Geometry: final body of the model. Coordinates: model frame, mm. A direction names the side the tool comes from. Give positions to 0.01 mm unless a question says otherwise; leave off trailing zeros. Write each loop counter-clockwise with the first axis right and the second up, starting at its lowest first coordinate (ties: lowest second). Pieces come first, ordered by that corner, then holes. Notation, with made-up numbers: (-15, 82) -> (0, 82) arc R32 cw to (0, 115) -> close; hole circle Ø3 at (17.5, -33). An arc over 180 degrees is marked (long way). Answer as a JSON object with one key per item and string values. Group by question number.
(1) Section query A-A on x = 6.75. Output: boundary loops of the cut face in (y, z), plus the area to 3 significant figures.
(2) Draft query along Y for faces 6 (the face through (12.32, -14.79, 61.76)), 7 (the face through (12, -6, 50)), 8 (the face through (12, -45, 140)). Return one class per face: +Y half, -Y half, draft (parallel to the pull), parting line (faces both ways), or undercut.
(3) Material intervals for probe 1 along Z at (x, y) = (13.5, -53.5); probe 2 along X at (y, z) = (-6, 33); probe 3 along Y at (x, z) = (12.5, 38.5), sorted ascending.
(4) Section query C-C on x = 22.5. Output: boundary loops of the cut face in (y, z), plus the area to 3 significant figures.
(5) Set-up query: faces 1 (the face through (6, -45, 110)), 2 (the face through (12, -53, 25)), 3 (the face through (12, 0, 26)), 4 (the face through (0, -37, 56)), 5 (the face through (12, -30, 105)). Return all of +Z, -Z, +X, -X, +Y, -Y with unobstructed straight access to the full face (end or side cutting, diameter ignored); none if empty.
(6) Contact query for flat-ended pins moving along their axis: pin 1 Ø12.5 at (x, z) = (17, 116.5) entering from +Y; pin 2 Ø7 at (x, y) = (12.5, -6) entering from +Z; pin 3 Ø8 at (x, y) = (2.5, -13) entering from +Z. Output: stop coordinate, or through.
(7) Section query B-B on y = -25. Output: boundary loops of the cut face in (x, z), plus the area to 3 significant figures.
(8) Section query D-D on y = -13. Output: boundary loops of the cut face in (x, z).
from build123d import *

# Parameters (mm, degrees)
F1_DEPTH = 25
F3_DEPTH = 50
F5_DEPTH = 60


with BuildPart() as f1:
    # F0 (on Right) → F1 (new body)
    with BuildSketch(Plane.YZ):
        with BuildLine():
            Line((-60, 0), (0, 0))
            Line((0, 0), (0, 53.749684))
            Line((0, 53.749684), (-30, 70))
            Line((-30, 70), (-30, 140))
            Line((-30, 140), (-60, 140))
            Line((-60, 140), (-60, 25))
            Line((-60, 25), (-45, 25))
            ThreePointArc((-45, 25), (-5.006255, 25.500156), (-44.974984, 24))
            Line((-44.974984, 24), (-60, 24))
            Line((-60, 24), (-60, 12))
            Line((-60, 12), (-60, 0))
        make_face()
    extrude(amount=F1_DEPTH)

    # F2 (on Top) → F3 (cut)
    with BuildSketch(Plane.XY):
        with BuildLine():
            ThreePointArc((12.5, -2), (9.671573, -8.828427), (16.5, -6))
            ThreePointArc((16.5, -6), (15.328427, -3.171573), (12.5, -2))
        make_face()
    extrude(amount=F3_DEPTH, mode=Mode.SUBTRACT)

    # F4 (on Front) → F5 (cut)
    with BuildSketch(Plane.XZ):
        Polygon((-7.744254, 110), (0, 110), (12.5, 110), (12.5, 122.5), (-7.744254, 122.5), align=None)
    extrude(amount=F5_DEPTH, mode=Mode.SUBTRACT)


solid = f1.part
Answer list:
{
 "1": {"outline": "(-60, 0) -> (0, 0) -> (0, 53.75) -> (-30, 70) -> (-30, 110) -> (-60, 110) -> (-60, 25) -> (-45, 25) arc R20 cw (long way) to (-44.97, 24) -> (-60, 24) -> close; (-60, 122.5) -> (-30, 122.5) -> (-30, 140) -> (-60, 140) -> close", "area": "4,410 mm2"},
 "2": {"face 6": "+Y half", "face 7": "undercut", "face 8": "draft"},
 "3": {"probe 1": "0 to 24, 25 to 140", "probe 2": "0 to 8.5, 16.5 to 25", "probe 3": "-60 to -39.76, -10.24 to -10, -2 to 0"},
 "4": {"outline": "(-60, 0) -> (0, 0) -> (0, 53.75) -> (-30, 70) -> (-30, 140) -> (-60, 140) -> (-60, 25) -> (-45, 25) arc R20 cw (long way) to (-44.97, 24) -> (-60, 24) -> close", "area": "4,780 mm2"},
 "5": {"face 1": "-X, +Y, -Y", "face 2": "+X, -X, -Y", "face 3": "+Z, -Z, +X, -X, +Y", "face 4": "+Z, -Z, -X, +Y, -Y", "face 5": "+Z, +X, -X, +Y"},
 "6": {"pin 1": "y = -30", "pin 2": "z = 58.9", "pin 3": "z = 62.96"},
 "7": {"outline": "(0, 0) -> (25, 0) -> (25, 5) -> (0, 5) -> close; (0, 45) -> (25, 45) -> (25, 67.29) -> (0, 67.29) -> close", "area": "682 mm2"},
 "8": {"outline": "(0, 0) -> (25, 0) -> (25, 9) -> (0, 9) -> close; (0, 41) -> (25, 41) -> (25, 60.79) -> (0, 60.79) -> close"}
}
